Geometry check sheet. Reference: drawing and pictorial views, mm from the part's lowest x, y, z. Coordinates: 2 decimals unless noted, no trailing zeros. Order: outer loops, then holes, each group sorted by start corner. A loop starts at its lowest first (then second) coordinate and runs counter-clockwise, first axis right, second up. Notation, with made-up numbers: (61.5, 0) -> (78.5, 0) arc R25 ccw to (78.5, 19) -> close; hole circle Ø7 at (1.5, -24.75). An arc over 180 degrees is marked (long way). Use CSV: the item, a comma, the result in double quotes. Start each with the question number.
1) Scan lines: line 1 along Y through (x, z) = (32, 0.25) (1 decimal); line 2 along Y through (x, z) = (30.5, 0.8) (1 decimal); line 3 along X through (y, z) = (38, 1.7) (1 decimal). Record each from-to range of solid material in increasing order.
2) Sectioned sample at B-B on y = 5. Record the boundary of the cut face in (x, z).
3) Sectioned sample at D-D on y = 31.5. Record the boundary of the cut face in (x, z).
4) Sectioned sample at C-C on z = 0.9. Give the number of separate pieces and of enclosed holes in the cut face, then the cut area to 3 significant figures.
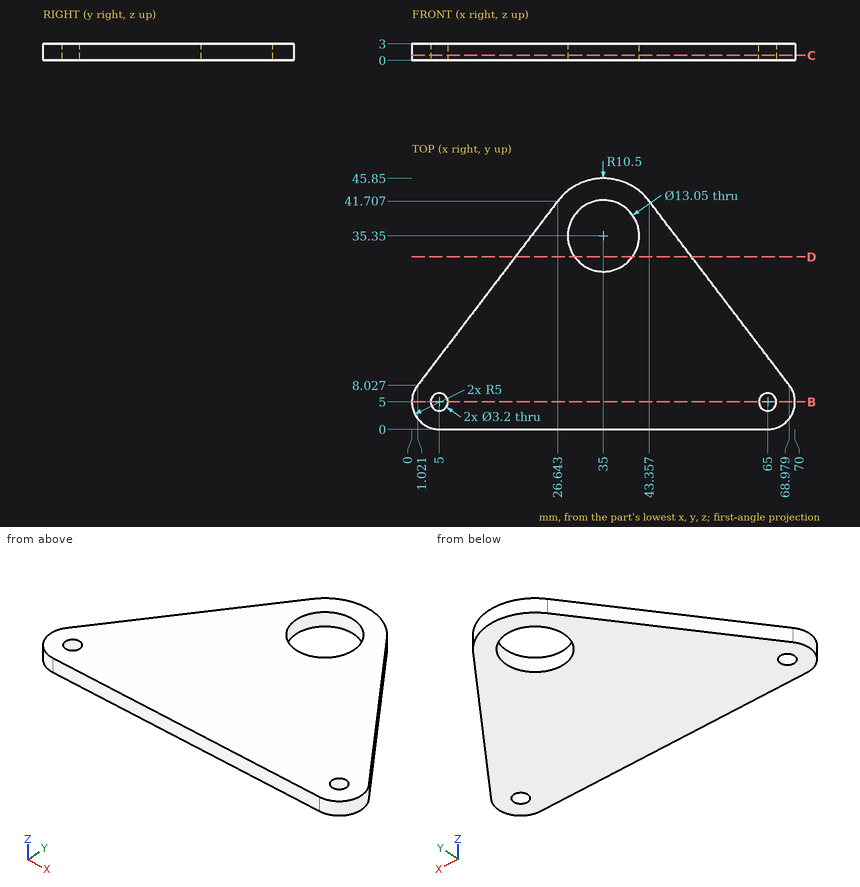
Answers follow:
1,line 1,"y = 0 to 29.6, 41.1 to 45.4"
1,line 2,"y = 0 to 30.6, 40.1 to 44.8"
1,line 3,"x = 23.8 to 29, 41 to 46.2"
2,outline,"(0, 0) -> (3.4, 0) -> (3.4, 3) -> (0, 3) -> close; (6.6, 0) -> (63.4, 0) -> (63.4, 3) -> (6.6, 3) -> close; (66.6, 0) -> (70, 0) -> (70, 3) -> (66.6, 3) -> close"
3,outline,"(18.88, 0) -> (29.73, 0) -> (29.73, 3) -> (18.88, 3) -> close; (40.27, 0) -> (51.12, 0) -> (51.12, 3) -> (40.27, 3) -> close"
4,separate pieces,"1"
4,enclosed holes,"3"
4,area,"1,870 mm²"
